Build history of the part. All positions in model axes, mm. A direction names the side the tool comes from. Round coordinates to 2 decimals unless told otherwise and drop trailing zeros. Write each loop counter-clockwise with the first axis right and the second up, starting at its lowest first coordinate (ties: lowest second). Pieces come first, ordered by that corner, then holes.
1) Saw through at D-D (y = 30). Write the cut outline in (x, z) (3 decimals).
2) Saw through at A-A (x = -30.48). Write the cut outline in (y, z).
3) Saw through at C-C (z = 6.35). Write the cut outline in (x, y), plus the area to 3 significant figures.
4) Saw through at B-B (y = 26). Write the cut outline in (x, z) (3 decimals).
5) Pull direction Z, two halves, no side cores. Call faces 1 (the flat face through (1, 29, 0)), 2 (the cylindrical face through (28.08, 29.1, 6.88)), 3 (the cylindrical face through (17.55, 27.28, 6.26)): +Z half, -Z half, draft (parallel to the pull), parting line (faces both ways), or undercut.
6) Flat gauge pins, fed straight in: pin 1 (3 mm diameter, centred on x = -30.48, z = 6.35, fed in from +Y); pin 2 (5.5 mm diameter, centred on x = 30.48, z = 6.35, fed in from -Y); pin 3 (3 mm diameter, centred on y = 26.5, z = 1.5, fed in from -X). Where does each tip first touch, or does it go through?
7) Wall check: probe 1 along X at (y, z) = (31.5, 6.35); probe 2 along X at (y, z) = (29.25, 7.5); probe 3 along X at (y, z) = (25.5, 2.5). Give the ranges that are in metal, low to high.
8) Which spindle directions (+Z, -Z, +X, -X, +Y, -Y) get a long thin tool onto all of the face, cutting with end or side? Do faces 4 (the flat face through (-3, 24.714, 6)), 5 (the flat face through (-41, 29, 9.525)). Say none if no direction does.
from build123d import *

# Parameters (mm, degrees)
BOSS_EXTRUDE1_DEPTH          = 12.7
SKETCH2_W                    = 3.175
SKETCH2_H                    = 8.89
BOSS_EXTRUDE2_DEPTH          = 6.35
F_10_0_1935_DIAMETER_HOLE1_D = 4.9149


with BuildPart() as part:
    # Sketch1 → Boss-Extrude1 (new body)
    with BuildSketch(Plane.XY):
        with BuildLine():
            Line((38.1, 33.6042), (38.1, 24.7142))
            Line((38.1, 24.7142), (22.561451151, 24.7142))
            ThreePointArc((22.561451151, 24.7142), (17.4625, 27.2796), (12.363548849, 24.7142))
            Line((12.363548849, 24.7142), (-12.363548849, 24.7142))
            ThreePointArc((-12.363548849, 24.7142), (-17.4625, 27.2796), (-22.561451151, 24.7142))
            Line((-22.561451151, 24.7142), (-38.1, 24.7142))
            Line((-38.1, 24.7142), (-38.1, 33.6042))
            Line((-38.1, 33.6042), (38.1, 33.6042))
        make_face()
    extrude(amount=BOSS_EXTRUDE1_DEPTH)

    # Sketch2 → Boss-Extrude2 (add)
    with BuildSketch(Plane.ZY.offset(38.1)):
        with Locations((11.1125, 29.1592)):
            Rectangle(SKETCH2_W, SKETCH2_H)
    extrude(amount=BOSS_EXTRUDE2_DEPTH)

    # #10 (0.1935) Diameter Hole1 (through all)
    with Locations(Plane(origin=(-30.48, 33.6042, 6.35), x_dir=(0, 0, 1), z_dir=(0, 1, 0))):
        with Locations((0, 0), (0, 30.48), (0, 60.96)):
            Hole(F_10_0_1935_DIAMETER_HOLE1_D / 2)


solid = part.part
Evaluation:
1. outline: (-44.45, 9.525) - (-38.1, 9.525) - (-38.1, 0) - (38.1, 0) - (38.1, 12.7) - (-44.45, 12.7) - close; hole circle Ø4.915 at (-30.48, 6.35); hole circle Ø4.915 at (0, 6.35); hole circle Ø4.915 at (30.48, 6.35)
2. outline: (24.71, 0) - (33.6, 0) - (33.6, 3.89) - (24.71, 3.89) - close; (24.71, 8.81) - (33.6, 8.81) - (33.6, 12.7) - (24.71, 12.7) - close
3. outline: (-38.1, 24.71) - (-32.94, 24.71) - (-32.94, 33.6) - (-38.1, 33.6) - close; (-28.02, 24.71) - (-22.56, 24.71) arc R6.35 cw to (-12.36, 24.71) - (-2.46, 24.71) - (-2.46, 33.6) - (-28.02, 33.6) - close; (2.46, 24.71) - (12.36, 24.71) arc R6.35 cw to (22.56, 24.71) - (28.02, 24.71) - (28.02, 33.6) - (2.46, 33.6) - close; (32.94, 24.71) - (38.1, 24.71) - (38.1, 33.6) - (32.94, 33.6) - close
3. area: 510 mm2
4. outline: (-44.45, 9.525) - (-38.1, 9.525) - (-38.1, 0) - (-21.285, 0) - (-21.285, 12.7) - (-44.45, 12.7) - close; (-13.64, 0) - (13.64, 0) - (13.64, 12.7) - (-13.64, 12.7) - close; (21.285, 0) - (38.1, 0) - (38.1, 12.7) - (21.285, 12.7) - close; hole circle Ø4.915 at (-30.48, 6.35); hole circle Ø4.915 at (0, 6.35); hole circle Ø4.915 at (30.48, 6.35)
5. face 1: -Z half
5. face 2: undercut
5. face 3: draft
6. pin 1: passes through
6. pin 2: stops at y = 24.71
6. pin 3: stops at x = -38.1
7. probe 1: x = -38.1 to -32.94, -28.02 to -2.46, 2.46 to 28.02, 32.94 to 38.1
7. probe 2: x = -38.1 to -32.65, -28.31 to -2.17, 2.17 to 28.31, 32.65 to 38.1
7. probe 3: x = -38.1 to -21.87, -13.05 to 13.05, 21.87 to 38.1
8. face 4: +Z, -Z, +X, -X, -Y
8. face 5: -Z, -X, +Y, -Y
